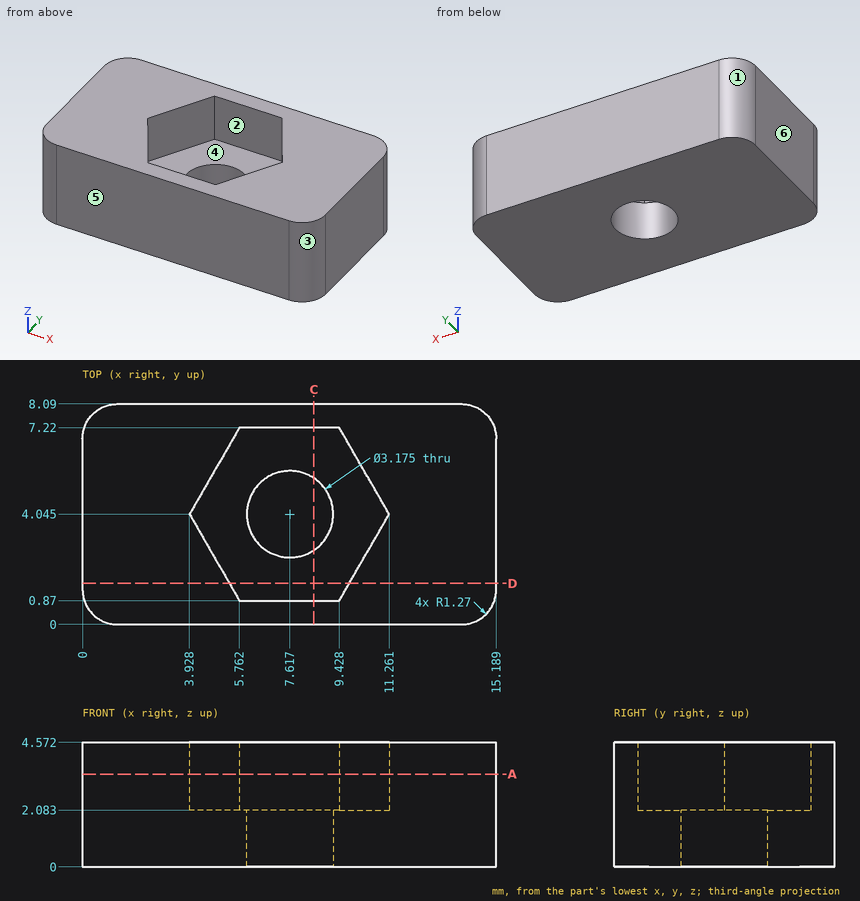
The figure shows three views and two pictorial views of one solid part (mm, origin at its lowest corner). Answer the questions. A direction names the side the tool comes from. Coordinates: 2 decimals unless noted, no trailing zeros. Order: outer loops, then holes, each group sorted by start corner. A loop starts at its lowest first (then second) coordinate and runs counter-clockwise, first axis right, second up. Notation, with made-up numbers: M -4,12 L 40,12 A31 cw 40,37 Z; hole C -22.5,11.25 d7. An arc over 180 degrees is marked long. Use CSV: the item, a comma, the result in double quotes.
1) A flat-ended cylindrical pin translates along its axis: pin 1 Ø1.9 at (x, y) = (7.62, 4.04) entering from -Z. Find the tip coordinate at first contact, or state that the pin passes through.
Worked out:
pin 1,"passes through"
2) Section A-A on z = 3.4 is taken. Write down the section's boundary in (x, y) (1 decimal).
Worked out:
outline,"M 0,1.3 A1.3 ccw 1.3,0 L 13.9,0 A1.3 ccw 15.2,1.3 L 15.2,6.8 A1.3 ccw 13.9,8.1 L 1.3,8.1 A1.3 ccw 0,6.8 Z; hole M 3.9,4 L 5.8,0.9 L 9.4,0.9 L 11.3,4 L 9.4,7.2 L 5.8,7.2 Z"
3) Determine the mould class of the marked faces 3, 4, 5 and 6 for opening direction X: released by +X, released by -X, zero draft, split by the parting line, or undercut.
Worked out:
face 3,"released by +X"
face 4,"undercut"
face 5,"zero draft"
face 6,"released by -X"
4) Section D-D on y = 1.5 is taken. Write down the section's boundary in (x, z).
Worked out:
outline,"M 0,0 L 15.19,0 L 15.19,4.57 L 9.79,4.57 L 9.79,2.08 L 5.4,2.08 L 5.4,4.57 L 0,4.57 Z"
5) Consider line 1 (Z direction, x = 10, y = 2); line 2 (Y direction, x = 6, z = 3.7); line 3 (X direction, y = 5, z = 2.3). Determine where each line is inside the solid, lowest interval first. Write a range as [from, to].
Worked out:
line 1,"z = [0, 2.08]"
line 2,"y = [0, 0.87], [7.22, 8.09]"
line 3,"x = [0, 4.48], [10.71, 15.19]"
6) Section C-C on x = 8.5 is taken. Write down the section's boundary in (y, z) (1 decimal).
Worked out:
outline,"M 0,0 L 2.7,0 L 2.7,2.1 L 0.9,2.1 L 0.9,4.6 L 0,4.6 Z; M 5.4,0 L 8.1,0 L 8.1,4.6 L 7.2,4.6 L 7.2,2.1 L 5.4,2.1 Z"
7) For the marked faces 1 and 2, determine the directions among +Z, -Z, +X, -X, +Y, -Y from which every point of the face is accessible in a straight line to the end or side of a thin tool.
Worked out:
face 1,"+Z, -Z, -X, +Y"
face 2,"+Z"
